Build history of the part. All positions in model axes, mm. Face numbers are marked on the shaded views. A direction names the side the tool comes from. Coordinates: 2 decimals unless noted, no trailing zeros. Order: outer loops, then holes, each group sorted by start corner. A loop starts at its lowest first (then second) coordinate and runs counter-clockwise, first axis right, second up. Notation, with made-up numbers: (-25, 21) - (2, 21) arc R15 cw to (2, 47) - close; hole circle Ø9 at (81, 44). An arc over 180 degrees is marked (long way). Return JSON: item names as keys, results as strings.
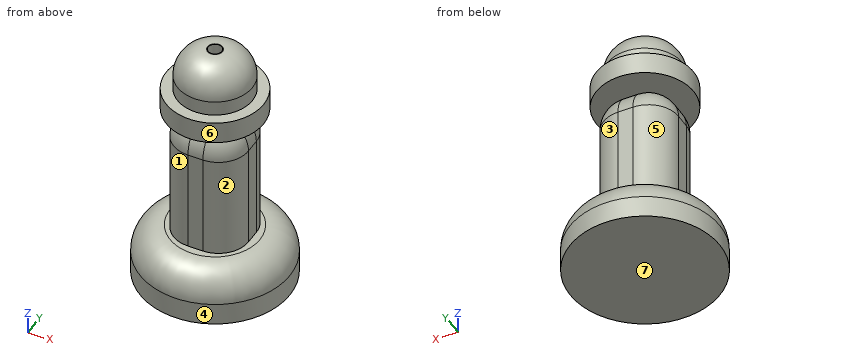
from build123d import *

# Parameters (mm, degrees)
F0_R         = 12.7
F1_DEPTH     = 8.89
F2_W         = 12.7
F2_H         = 12.7
F3_DEPTH     = 31.75
F4_R         = 5.08
F5_T1_DEPTH  = 17.78
F5_S5_W      = 5.08
F5_S5_H      = 5.08
F5_T6_DEPTH  = 5.08
F5_S11_W     = 5.08
F5_S11_H     = 5.08
F5_T12_DEPTH = 5.08
F5_S17_W     = 5.08
F5_S17_H     = 5.08
F5_T18_DEPTH = 5.08
F5_S23_W     = 5.08
F5_S23_H     = 5.08
F5_T24_DEPTH = 5.08
F6_R         = 8.255
F7_DEPTH     = 3.81
F8_R         = 6.35
F9_DEPTH     = 7.62
F10_R        = 5.08
F12_D        = 2.286
F12_DEPTH    = 12.7
F12_TIP      = 0.6867836875
F13_R        = 5.08


# Not quite as in the source:
# - a fillet or chamfer that OpenCascade refuses, or shapes differently, is made with other operations: its cross-section is extruded or revolved along the edge and cut away or added


with BuildPart() as f1:
    # F0 (on Top) → F1 (new body)
    with BuildSketch(Plane.XY):
        Circle(F0_R)
    extrude(amount=F1_DEPTH)

    # F2 (on Top) → F3 (join)
    with BuildSketch(Plane.XY):
        Rectangle(F2_W, F2_H)
    extrude(amount=F3_DEPTH)

    # F4
    f4_edges = [f1.edges().sort_by_distance(p)[0] for p in [
        (6.35, 0, 31.75),
        (0, -6.35, 31.75),
        (-6.35, 0, 31.75),
        (0, 6.35, 31.75),
    ]]
    fillet(f4_edges, radius=F4_R)

    # F5: fillet of radius 5.08 on 4 edges, made by hand

    # F5_s2 → F5_t1 (cut)
    with BuildSketch(Plane.XY.offset(8.89)):
        with BuildLine():
            ThreePointArc((1.27, -6.35), (4.8621024484, -4.8621024484), (6.35, -1.27))
            Line((6.35, -1.27), (6.35, -6.35))
            Line((6.35, -6.35), (1.27, -6.35))
        make_face()
        with BuildLine():
            ThreePointArc((-6.35, -1.27), (-4.8621024484, -4.8621024484), (-1.27, -6.35))
            Line((-1.27, -6.35), (-6.35, -6.35))
            Line((-6.35, -6.35), (-6.35, -1.27))
        make_face()
        with BuildLine():
            ThreePointArc((-6.35, 1.27), (-4.8621024484, 4.8621024484), (-1.27, 6.35))
            Line((-1.27, 6.35), (-6.35, 6.35))
            Line((-6.35, 6.35), (-6.35, 1.27))
        make_face()
        with BuildLine():
            ThreePointArc((1.27, 6.35), (4.8621024484, 4.8621024484), (6.35, 1.27))
            Line((6.35, 1.27), (6.35, 6.35))
            Line((6.35, 6.35), (1.27, 6.35))
        make_face()
    extrude(amount=F5_T1_DEPTH, mode=Mode.SUBTRACT)


with BuildPart() as f5_tool4:
    # F5_s5 → F5_t6 (new body)
    with BuildSketch(Plane.XZ.offset(-1.27)):
        with Locations((3.81, 29.21)):
            Rectangle(F5_S5_W, F5_S5_H)
    extrude(amount=-F5_T6_DEPTH)

    # F5_s7 → F5_t8 (revolve, cut)
    with BuildSketch(Plane(origin=(1.27, 1.27, 26.67), x_dir=(-0.7071067812, 0, -0.7071067812), z_dir=(0.7071067812, 0, -0.7071067812))):
        with BuildLine():
            ThreePointArc((0, -5.08), (5.08, 0), (0, 5.08))
            Line((0, 5.08), (0, -5.08))
        make_face()
    revolve(axis=Axis((1.27, 1.27, 26.67), (0, 1, 0)), mode=Mode.SUBTRACT)


with BuildPart() as f1_1:
    add(f1.part)

    # F5_t3: cut F5_tool4
    add(f5_tool4.part, mode=Mode.SUBTRACT)


with BuildPart() as f5_tool10:
    # F5_s11 → F5_t12 (new body)
    with BuildSketch(Plane.YZ.offset(-1.27)):
        with Locations((3.81, 29.21)):
            Rectangle(F5_S11_W, F5_S11_H)
    extrude(amount=-F5_T12_DEPTH)

    # F5_s13 → F5_t14 (revolve, cut)
    with BuildSketch(Plane(origin=(-1.27, 1.27, 26.67), x_dir=(0, -0.7071067812, -0.7071067812), z_dir=(0, 0.7071067812, -0.7071067812))):
        with BuildLine():
            ThreePointArc((0, -5.08), (5.08, 0), (0, 5.08))
            Line((0, 5.08), (0, -5.08))
        make_face()
    revolve(axis=Axis((-1.27, 1.27, 26.67), (-1, 0, 0)), mode=Mode.SUBTRACT)


with BuildPart() as f1_2:
    add(f1_1.part)

    # F5_t9: cut F5_tool10
    add(f5_tool10.part, mode=Mode.SUBTRACT)


with BuildPart() as f5_tool16:
    # F5_s17 → F5_t18 (new body)
    with BuildSketch(Plane.YZ.offset(-1.27)):
        with Locations((-3.81, 29.21)):
            Rectangle(F5_S17_W, F5_S17_H)
    extrude(amount=-F5_T18_DEPTH)

    # F5_s19 → F5_t20 (revolve, cut)
    with BuildSketch(Plane(origin=(-1.27, -1.27, 26.67), x_dir=(0, 0.7071067812, -0.7071067812), z_dir=(0, 0.7071067812, 0.7071067812))):
        with BuildLine():
            ThreePointArc((0, -5.08), (5.08, 0), (0, 5.08))
            Line((0, 5.08), (0, -5.08))
        make_face()
    revolve(axis=Axis((-1.27, -1.27, 26.67), (-1, 0, 0)), mode=Mode.SUBTRACT)


with BuildPart() as f1_3:
    add(f1_2.part)

    # F5_t15: cut F5_tool16
    add(f5_tool16.part, mode=Mode.SUBTRACT)


with BuildPart() as f5_tool22:
    # F5_s23 → F5_t24 (new body)
    with BuildSketch(Plane.XZ.offset(1.27)):
        with Locations((3.81, 29.21)):
            Rectangle(F5_S23_W, F5_S23_H)
    extrude(amount=F5_T24_DEPTH)

    # F5_s25 → F5_t26 (revolve, cut)
    with BuildSketch(Plane(origin=(1.27, -1.27, 26.67), x_dir=(-0.7071067812, 0, -0.7071067812), z_dir=(-0.7071067812, 0, 0.7071067812))):
        with BuildLine():
            ThreePointArc((0, -5.08), (5.08, 0), (0, 5.08))
            Line((0, 5.08), (0, -5.08))
        make_face()
    revolve(axis=Axis((1.27, -1.27, 26.67), (0, -1, 0)), mode=Mode.SUBTRACT)


with BuildPart() as f1_4:
    add(f1_3.part)

    # F5_t21: cut F5_tool22
    add(f5_tool22.part, mode=Mode.SUBTRACT)

    # F6 (on face) → F7 (join)
    with BuildSketch(Plane.XY.offset(31.75)):
        Circle(F6_R)
    extrude(amount=F7_DEPTH)

    # F8 (on face) → F9 (join)
    with BuildSketch(Plane.XY.offset(35.56)):
        Circle(F8_R)
    extrude(amount=F9_DEPTH)

    # F10
    f10_edges = [f1_4.edges().sort_by_distance(p)[0] for p in [
        (-6.35, 0, 43.18),
    ]]
    fillet(f10_edges, radius=F10_R)

    # F12
    with Locations(Plane.XY.offset(43.18)):
        with Locations((0, 0)):
            Hole(F12_D / 2, depth=F12_DEPTH)
            with Locations((0, 0, -(F12_DEPTH + F12_TIP / 2))):  # 118° drill point
                Cone(0, F12_D / 2, F12_TIP, mode=Mode.SUBTRACT)

    # F13
    f13_edges = [f1_4.edges().sort_by_distance(p)[0] for p in [
        (-12.7, 0, 8.89),
    ]]
    fillet(f13_edges, radius=F13_R)


solid = f1_4.part
1. Cut at B-B on z = 32.5. Give the cut face in (x, y) (3 decimals), plus the area to 3 significant figures.
Check values:
{"outline": "circle Ø16.51 at (0, 0); hole circle Ø2.286 at (0, 0)", "area": "210 mm²"}
2. Probe L1, parallel to Y at x = 0, z = 35 (3 decimals); L2, parallel to Z at x = -4, y = -2.5; L3, parallel to Z at x = -1, y = -4.25. List the from-to ranges inside material, lowest first.
Check values:
{"L1": "-8.255 to -1.143, 1.143 to 8.255", "L2": "0 to 30.77, 31.75 to 41.83", "L3": "0 to 30.78, 31.75 to 42.13"}
3. Cut at C-C on z = 27.5. Give the cut face in (x, y).
Check values:
{"outline": "(-6.28, -1.27) arc R5.01 ccw to (-1.27, -6.28) - (1.27, -6.28) arc R5.01 ccw to (6.28, -1.27) - (6.28, 1.27) arc R5.01 ccw to (1.27, 6.28) - (-1.27, 6.28) arc R5.01 ccw to (-6.28, 1.27) - close"}
4. Tool access for the marked faces 1, 2, 3 and 4: list every direction of +Z, -Z, +X, -X, +Y, -Y with a clear straight run to the whole face (end or side of a thin tool).
Check values:
{"face 1": "-X, -Y", "face 2": "+X, -Y", "face 3": "+X, +Y", "face 4": "+Z, -Z"}
5. Cut at A-A on z = 16.5. Give the cut face in (x, y).
Check values:
{"outline": "(-6.35, -1.27) arc R5.08 ccw to (-1.27, -6.35) - (1.27, -6.35) arc R5.08 ccw to (6.35, -1.27) - (6.35, 1.27) arc R5.08 ccw to (1.27, 6.35) - (-1.27, 6.35) arc R5.08 ccw to (-6.35, 1.27) - close"}
6. Drop flat-ended pins along their axis: pin 1 (2 mm diameter, centred on x = 0.5, z = 17, fed in from -Y); pin 2 (5 mm diameter, centred on x = 1.5, z = 18.5, fed in from +Y); pin 3 (12 mm diameter, centred on x = -1, y = -1.5, fed in from +Z); pin 4 (8 mm diameter, centred on y = -3.5, z = 7.5, fed in from +X). Give the stop position or say it passes through.
Check values:
{"pin 1": "y = -6.35", "pin 2": "y = 6.35", "pin 3": "z = 43.18", "pin 4": "x = 12.63"}
7. Mould opens along Z. For the marked faces 5, 6 and 7 say: pulls with the +Z half, pulls with the -Z half, needs draft (parallel to the pull), parting line crosses it, or undercut.
Check values:
{"face 5": "undercut", "face 6": "needs draft", "face 7": "pulls with the -Z half"}
